Model file for the job. Use its own axes, mm. Face numbers are marked on the shaded views. Coordinates: 2 decimals unless noted, no trailing zeros. Order: outer loops, then holes, each group sorted by start corner. A loop starts at its lowest first (then second) coordinate and runs counter-clockwise, first axis right, second up. Notation, with made-up numbers: (45, 36.5) -> (66, 36.5) arc R12 ccw to (66, 50.5) -> close; hole circle Ø8 at (-14.5, 8.25). An arc over 180 degrees is marked (long way). Return JSON: item names as keys, results as strings. Group by question number.
1) Cut at A-A (y = -67.5). Write the cut outline in (x, z).
2) Cut at B-B (z = 17). Write the cut outline in (x, y), and give its area (3 significant figures).
3) Cut at C-C (x = 48). Write the cut outline in (y, z), and give its area (3 significant figures).
4) Cut at D-D (x = 61). Write the cut outline in (y, z).
5) Probe line 1 (Y direction, x = 34, z = 18.5); line 2 (X direction, y = -12.5, z = 66); line 3 (X direction, y = -14, z = 63.5). List the from-to ranges inside material, lowest first.
6) Flat gauge pins, fed straight in: pin 1 (2 mm diameter, centred on x = 5.5, y = -92.5, fed in from -Z); pin 2 (2.5 mm diameter, centred on y = -38, z = 10.5, fed in from -X); pin 3 (1.5 mm diameter, centred on x = 17, y = -20, fed in from -Z). Where does each tip first touch, or does it go through?
7) Pull direction X, two halves, no side cores. Call the marked faces 1, 2 and 3: +X half, -X half, draft (parallel to the pull), parting line (faces both ways), or undercut.
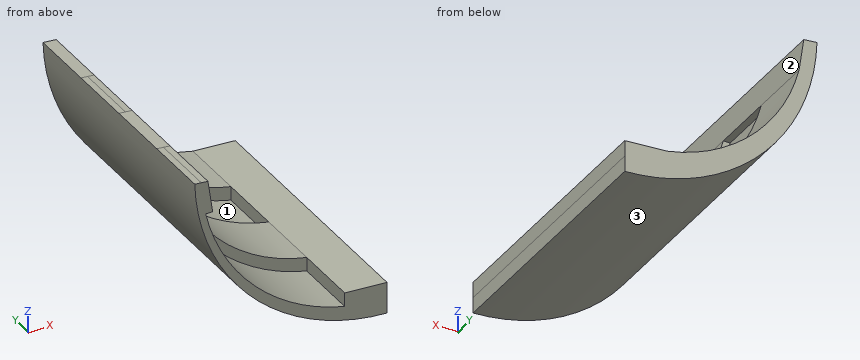
from build123d import *

# Parameters (mm, degrees)
F1_DEPTH = 76.2
F2_DEPTH = 50.8
F4_DEPTH = 50.8
F5_DEPTH = 25.4
F6_DEPTH = 50.8


with BuildPart() as f1:
    # F0 (on Front) → F1 (new body)
    with BuildSketch(Plane.XZ):
        with BuildLine():
            Line((5.060865, 73.516467), (0, 73.956974))
            ThreePointArc((0, 73.956974), (22.2398, 22.393389), (73.736869, 0))
            Line((73.736869, 0), (73.738756, 12.0904))
            ThreePointArc((73.738756, 12.0904), (26.455464, 28.330906), (5.060865, 73.516467))
        make_face()
    extrude(amount=F1_DEPTH)

    # F0 (on Front) → F2 (cut)
    with BuildSketch(Plane.XZ):
        with BuildLine():
            Line((5.060865, 73.516467), (0, 73.956974))
            ThreePointArc((0, 73.956974), (22.2398, 22.393389), (73.736869, 0))
            Line((73.736869, 0), (73.738756, 12.0904))
            ThreePointArc((73.738756, 12.0904), (26.455464, 28.330906), (5.060865, 73.516467))
        make_face()
    extrude(amount=F2_DEPTH, mode=Mode.SUBTRACT)

    # F3 (on face) → F4 (join)
    with BuildSketch(Plane(origin=(0, -50.8, 0), x_dir=(-1, 0, 0), z_dir=(0, 1, 0))):
        with BuildLine():
            Line((-73.738756, 12.0904), (-73.737813, 6.0452))
            ThreePointArc((-73.737813, 6.0452), (-65.578858, 6.40406), (-57.516672, 7.707316))
            Line((-57.516672, 7.707316), (-57.516672, 13.041316))
            Line((-57.516672, 13.041316), (-73.738756, 12.0904))
        make_face()
        with BuildLine():
            ThreePointArc((-57.516672, 7.707316), (-65.578858, 6.40406), (-73.737813, 6.0452))
            Line((-73.737813, 6.0452), (-73.736869, 0))
            ThreePointArc((-73.736869, 0), (-22.206337, 22.360026), (0, 73.956974))
            Line((0, 73.956974), (-2.530432, 73.73672))
            ThreePointArc((-2.530432, 73.73672), (-3.061646, 67.302687), (-4.181222, 60.94458))
            ThreePointArc((-4.181222, 60.94458), (-23.10727, 26.569993), (-57.516672, 7.707316))
        make_face()
        with BuildLine():
            Line((-6.860218, 60.94458), (-4.181222, 60.94458))
            ThreePointArc((-4.181222, 60.94458), (-3.061646, 67.302687), (-2.530432, 73.73672))
            Line((-2.530432, 73.73672), (-5.060865, 73.516467))
            Line((-5.060865, 73.516467), (-6.860218, 60.94458))
        make_face()
    extrude(amount=F4_DEPTH)

    # F0 (on Front) → F5 (join)
    with BuildSketch(Plane.XZ):
        with BuildLine():
            Line((5.060865, 73.516467), (0, 73.956974))
            ThreePointArc((0, 73.956974), (22.2398, 22.393389), (73.736869, 0))
            Line((73.736869, 0), (73.738756, 12.0904))
            ThreePointArc((73.738756, 12.0904), (26.455464, 28.330906), (5.060865, 73.516467))
        make_face()
    extrude(amount=F5_DEPTH)

    # F3 (on face) → F6 (join)
    with BuildSketch(Plane(origin=(0, -50.8, 0), x_dir=(-1, 0, 0), z_dir=(0, 1, 0))):
        with BuildLine():
            Line((-73.738756, 12.0904), (-73.737813, 6.0452))
            ThreePointArc((-73.737813, 6.0452), (-65.578858, 6.40406), (-57.516672, 7.707316))
            Line((-57.516672, 7.707316), (-57.516672, 13.041316))
            Line((-57.516672, 13.041316), (-73.738756, 12.0904))
        make_face()
        with BuildLine():
            ThreePointArc((-57.516672, 7.707316), (-65.578858, 6.40406), (-73.737813, 6.0452))
            Line((-73.737813, 6.0452), (-73.736869, 0))
            ThreePointArc((-73.736869, 0), (-22.206337, 22.360026), (0, 73.956974))
            Line((0, 73.956974), (-2.530432, 73.73672))
            ThreePointArc((-2.530432, 73.73672), (-3.061646, 67.302687), (-4.181222, 60.94458))
            ThreePointArc((-4.181222, 60.94458), (-23.10727, 26.569993), (-57.516672, 7.707316))
        make_face()
        with BuildLine():
            Line((-6.860218, 60.94458), (-4.181222, 60.94458))
            ThreePointArc((-4.181222, 60.94458), (-3.061646, 67.302687), (-2.530432, 73.73672))
            Line((-2.530432, 73.73672), (-5.060865, 73.516467))
            Line((-5.060865, 73.516467), (-6.860218, 60.94458))
        make_face()
    extrude(amount=-F6_DEPTH)


solid = f1.part
Answers below:
{
 "1": {"outline": "(0, 73.96) arc R76.2 ccw to (73.74, 0) -> (73.74, 6.05) -> (73.74, 12.09) -> (57.52, 13.04) arc R64.36 cw to (6.86, 60.94) -> (5.06, 73.52) -> close"},
 "2": {"outline": "(28.14, -101.6) -> (35.06, -101.6) -> (35.06, -76.2) -> (44.35, -76.2) -> (44.35, -50.8) -> (35.06, -50.8) -> (35.06, -25.4) -> (44.35, -25.4) -> (44.35, 0) -> (28.14, 0) -> close", "area": "1,170 mm^2"},
 "3": {"outline": "(-101.6, 5.36) -> (0, 5.36) -> (0, 15.59) -> (-25.4, 15.59) -> (-25.4, 10.54) -> (-50.8, 10.54) -> (-50.8, 15.59) -> (-76.2, 15.59) -> (-76.2, 10.54) -> (-101.6, 10.54) -> close", "area": "783 mm^2"},
 "4": {"outline": "(-101.6, 1.49) -> (0, 1.49) -> (0, 12.84) -> (-101.6, 12.84) -> close"},
 "5": {"line 1": "y = -76.2 to -50.8, -25.4 to 0", "line 2": "x = 0.65 to 6.14", "line 3": "x = 1.03 to 6.49"},
 "6": {"pin 1": "stops at z = 45.29", "pin 2": "stops at x = 35.45", "pin 3": "stops at z = 27.24"},
 "7": {"face 1": "undercut", "face 2": "+X half", "face 3": "-X half"}
}
